Geometry: final body of the model. Coordinates: model frame, mm. A direction names the side the tool comes from. Give positions to 0.01 mm unless a question says otherwise; leave off trailing zeros. Order: outer loops, then holes, each group sorted by start corner. A loop starts at its lowest first (then second) coordinate and runs counter-clockwise, first axis right, second up. Notation, with made-up numbers: (51.5, 33.25) - (87.5, 33.25) arc R12 ccw to (87.5, 56.25) - close; hole circle Ø5 at (42, 15.5). An arc over 180 degrees is marked (long way). One line per question, with ' | ' between items. Start each with the question number.
from build123d import *

# Parameters (mm, degrees)
SKETCH1_W                = 20
SKETCH1_H                = 40
BOSS_EXTRUDE1_DEPTH      = 9
BOSS_EXTRUDE1_DEPTH_BACK = 26
SKETCH2_R                = 2.54
BOSS_EXTRUDE2_DEPTH      = 7.33
SKETCH3_W                = 8.88
SKETCH3_H                = 45.08
BOSS_EXTRUDE3_DEPTH      = 1.97
SKETCH6_W                = 20
SKETCH6_H                = 10
BOSS_EXTRUDE5_DEPTH      = 2
SKETCH8_R                = 2.15
CUT_EXTRUDE1_DEPTH       = 5.159375


with BuildPart() as part:
    # Sketch1 → Boss-Extrude1 (new body, two sides)
    with BuildSketch(Plane(origin=(0, 0, 0), x_dir=(1, 0, 0), z_dir=(0, 1, 0))) as boss_extrude1_sk:
        Rectangle(SKETCH1_W, SKETCH1_H)
    extrude(amount=BOSS_EXTRUDE1_DEPTH)
    extrude(boss_extrude1_sk.sketch, amount=-BOSS_EXTRUDE1_DEPTH_BACK)

    # Sketch2 → Boss-Extrude2 (add)
    with BuildSketch(Plane(origin=(0, 9, 0), x_dir=(1, 0, 0), z_dir=(0, 1, 0))):
        with Locations((0, 13.65)):
            Circle(SKETCH2_R)
    extrude(amount=BOSS_EXTRUDE2_DEPTH)

    # Sketch3 → Boss-Extrude3 (add)
    with BuildSketch(Plane(origin=(0, 16.33, 0), x_dir=(1, 0, 0), z_dir=(0, 1, 0))):
        with Locations((0, 13.65)):
            Rectangle(SKETCH3_W, SKETCH3_H)
    extrude(amount=BOSS_EXTRUDE3_DEPTH)

    # Sketch6 → Boss-Extrude5 (add)
    with BuildSketch(Plane(origin=(0, 0, 0), x_dir=(1, 0, 0), z_dir=(0, 1, 0))):
        with Locations((0, -25)):
            Rectangle(SKETCH6_W, SKETCH6_H)
        with Locations((0, 25)):
            Rectangle(SKETCH6_W, SKETCH6_H)
    extrude(amount=BOSS_EXTRUDE5_DEPTH)

    # Sketch8 → Cut-Extrude1 (cut)
    with BuildSketch(Plane(origin=(0, 0, 0), x_dir=(1, 0, 0), z_dir=(0, 1, 0))):
        with Locations((5.055, -24.285)):
            Circle(SKETCH8_R)
        with Locations((-5.055, -24.285)):
            Circle(SKETCH8_R)
        with Locations((5.055, 24.285)):
            Circle(SKETCH8_R)
        with Locations((-5.055, 24.285)):
            Circle(SKETCH8_R)
    extrude(amount=CUT_EXTRUDE1_DEPTH, mode=Mode.SUBTRACT)


solid = part.part
(1) Cut plane D-D, the plane y = 11. Return the cut outline in (x, z).
(2) Access query for faces 4 (the flat face through (0, 0, 25)), 5 (the flat face through (0, 2, -25)), 6 (the flat face through (0, 0, -25)). Directions: +Z, -Z, +X, -X, +Y, -Y. A direction counts if a zero-diameter tool reaches every point of the face in a straight line with its end or side. Return the directions, or none.
(3) Pull-direction query (Z, two-part tool) for faces 1 (the cylindrical face through (4.775, 0.986, 22.153)), 2 (the cylindrical face through (-0.55, 12.61, -11.17)), 3 (the flat face through (4.44, 17, -13)); classes: +Z half, -Z half, draft (parallel to the pull), parting line (faces both ways), or undercut.
(4) Cut plane C-C, the plane x = 8.25. Return the cut outline in (y, z), plus the area to 3 significant figures.
(5) Material intervals for line 1 along Y through (x, z) = (4, -5.5); line 2 along Y through (x, z) = (7.5, -20.5); line 3 along Z through (x, y) = (3, -13), sorted ascending. Write a range as from..to.
(6) Contact query for flat-ended pins moving along their axis: P1, Ø5.5, axis at x = 4.5, y = 5.5, coming from the +Z side; P2, Ø3.5, axis at x = 5.055, z = -24.285, coming from the -Y side; P3, Ø8, axis at x = -4.5, z = 26, coming from the -Y side; P4, Ø3.5, axis at x = -5.055, z = 24.285, coming from the +Y side. Output: stop coordinate, or through.
(7) Cut plane A-A, the plane z = -5. Return the cut outline in (x, y), plus the area to 3 significant figures.
(8) Cut plane B-B, the plane z = 23.5. Return the cut outline in (x, y), plus the area to 3 significant figures.
Results are:
1) outline: circle Ø5.08 at (0, -13.65)
2) face 4: +Z, +X, -X, -Y | face 5: -Z, +X, -X | face 6: -Z, +X, -X, -Y
3) face 1: undercut | face 2: parting line | face 3: draft
4) outline: (-26, -20) - (0, -20) - (0, -30) - (2, -30) - (2, -20) - (9, -20) - (9, 20) - (2, 20) - (2, 30) - (0, 30) - (0, 20) - (-26, 20) - close | area: 1,440 mm2
5) line 1: -26..9, 16.33..18.3 | line 2: 0..2 | line 3: -20..20
6) P1: z = 20 | P2: y = 16.33 | P3: y = 0 | P4: through
7) outline: (-10, -26) - (10, -26) - (10, 9) - (-10, 9) - close; (-4.44, 16.33) - (4.44, 16.33) - (4.44, 18.3) - (-4.44, 18.3) - close | area: 717 mm2
8) outline: (-10, 0) - (-7.06, 0) - (-7.06, 2) - (-10, 2) - close; (-3.05, 0) - (3.05, 0) - (3.05, 2) - (-3.05, 2) - close; (7.06, 0) - (10, 0) - (10, 2) - (7.06, 2) - close | area: 24.0 mm2
